from build123d import *

# Parameters (mm, degrees)
EXTRUDE_1_DEPTH      = 406.5
EXTRUDE_1_DEPTH_BACK = 406.5


with BuildPart() as part:
    # 草图1 → 凸台-拉伸1 (new, two sides: drawn at the far end of the back side and taken through both)
    with BuildSketch(Plane.XY.offset(-EXTRUDE_1_DEPTH_BACK)):
        with BuildLine():
            Line((24.75, 1), (24.75, 5.5))
            ThreePointArc((24.75, 5.5), (24.457106781, 6.207106781), (23.75, 6.5))
            Line((23.75, 6.5), (18.5, 6.5))
            Line((18.5, 6.5), (13.25, 6.5))
            ThreePointArc((13.25, 6.5), (12.542893219, 6.207106781), (12.25, 5.5))
            Line((12.25, 5.5), (12.25, 1))
            Line((12.25, 1), (1.35, 1))
            Line((1.35, 1), (1.35, 18))
            ThreePointArc((1.35, 18), (1.935786438, 19.414213562), (3.35, 20))
            Line((3.35, 20), (4.15, 20))
            ThreePointArc((4.15, 20), (4.503553391, 20.146446609), (4.65, 20.5))
            Line((4.65, 20.5), (4.65, 21))
            ThreePointArc((4.65, 21), (4.357106781, 21.707106781), (3.65, 22))
            Line((3.65, 22), (0.05, 22))
            Line((0.05, 22), (0.05, 27.351174762))
            Line((0.05, 27.351174762), (0.25, 27.351174762))
            Line((0.25, 27.351174762), (0.25, 32.3))
            Line((0.25, 32.3), (3.65, 32.3))
            Line((3.65, 32.3), (3.65, 26.3))
            ThreePointArc((3.65, 26.3), (4.15, 25.8), (4.65, 26.3))
            Line((4.65, 26.3), (4.65, 33.8))
            ThreePointArc((4.65, 33.8), (4.503553391, 34.153553391), (4.15, 34.3))
            Line((4.15, 34.3), (-0.35, 34.3))
            ThreePointArc((-0.35, 34.3), (-0.703553391, 34.153553391), (-0.85, 33.8))
            Line((-0.85, 33.8), (-0.85, 27.351174762))
            Line((-0.85, 27.351174762), (-1.35, 27.351174762))
            Line((-1.35, 27.351174762), (-1.35, 20.450932326))
            ThreePointArc((-1.35, 20.450932326), (-0.954594155, 19.496338171), (0, 19.100932326))
            Line((0, 19.100932326), (0, 1))
            ThreePointArc((0, 1), (0.292893219, 0.292893219), (1, 0))
            Line((1, 0), (15.25, 0))
            ThreePointArc((15.25, 0), (15.75, 0.5), (15.25, 1))
            Line((15.25, 1), (13.25, 1))
            Line((13.25, 1), (13.25, 5.5))
            Line((13.25, 5.5), (18.5, 5.5))
            Line((18.5, 5.5), (23.75, 5.5))
            Line((23.75, 5.5), (23.75, 1))
            Line((23.75, 1), (21.75, 1))
            ThreePointArc((21.75, 1), (21.25, 0.5), (21.75, 0))
            Line((21.75, 0), (36, 0))
            ThreePointArc((36, 0), (36.707106781, 0.292893219), (37, 1))
            Line((37, 1), (37, 19.100932326))
            ThreePointArc((37, 19.100932326), (37.954594155, 19.496338171), (38.35, 20.450932326))
            Line((38.35, 20.450932326), (38.35, 27.351174762))
            Line((38.35, 27.351174762), (37.85, 27.351174762))
            Line((37.85, 27.351174762), (37.85, 33.8))
            ThreePointArc((37.85, 33.8), (37.703553391, 34.153553391), (37.35, 34.3))
            Line((37.35, 34.3), (32.85, 34.3))
            ThreePointArc((32.85, 34.3), (32.496446609, 34.153553391), (32.35, 33.8))
            Line((32.35, 33.8), (32.35, 26.3))
            ThreePointArc((32.35, 26.3), (32.85, 25.8), (33.35, 26.3))
            Line((33.35, 26.3), (33.35, 32.3))
            Line((33.35, 32.3), (36.75, 32.3))
            Line((36.75, 32.3), (36.75, 27.351174762))
            Line((36.75, 27.351174762), (36.95, 27.351174762))
            Line((36.95, 27.351174762), (36.95, 22))
            Line((36.95, 22), (33.35, 22))
            ThreePointArc((33.35, 22), (32.642893219, 21.707106781), (32.35, 21))
            Line((32.35, 21), (32.35, 20.5))
            ThreePointArc((32.35, 20.5), (32.496446609, 20.146446609), (32.85, 20))
            Line((32.85, 20), (33.65, 20))
            ThreePointArc((33.65, 20), (35.064213562, 19.414213562), (35.65, 18))
            Line((35.65, 18), (35.65, 1))
            Line((35.65, 1), (24.75, 1))
        make_face()
    extrude(amount=EXTRUDE_1_DEPTH + EXTRUDE_1_DEPTH_BACK)


solid = part.part
The listing builds one solid part. Answer for the finished solid, in the listing's coordinates (mm). A direction names the side the tool comes from. Give positions to 0.01 mm unless a question says otherwise; leave off trailing zeros. Answer as CSV lines item,"result".
Item 1: Given pin 1 Ø4 at (x, z) = (21.5, 150) entering from +Y; pin 2 Ø3 at (x, z) = (18, 6.5) entering from -Y; pin 3 Ø6.5 at (y, z) = (29, 123) entering from -X; pin 4 Ø1 at (y, z) = (29.5, -244.5) entering from -X, each flat-ended and moving along its own axis, determine where each tip first touches the part or whether it passes through.
Values follow:
pin 1,"stops at y = 6.5"
pin 2,"stops at y = 5.5"
pin 3,"stops at x = -1.35"
pin 4,"stops at x = -0.85"
Item 2: The mould has two halves that part along X. Classify faces 1 (the flat face through (29, 0, -6)), 2 (the flat face through (37, 10, -6)), 3 (the flat face through (35.65, 10, -6)): released by +X, released by -X, zero draft, split by the parting line, or undercut.
Values follow:
face 1,"zero draft"
face 2,"released by +X"
face 3,"undercut"
Item 3: Straight lines are drawn through the part: line 1 along Y through (x, z) = (4, -225.5); line 2 along X through (y, z) = (27, -60.5); line 3 along X through (y, z) = (6, 369). For each, find the intervals that lie inside material, in ascending order. Write a range as [from, to].
Values follow:
line 1,"y = [0, 1], [20, 21.94], [25.82, 34.3]"
line 2,"x = [-1.35, 0.05], [3.65, 4.65], [32.35, 33.35], [36.95, 38.35]"
line 3,"x = [0, 1.35], [12.38, 24.62], [35.65, 37]"
Item 4: Which of the six approach directions +Z, -Z, +X, -X, +Y, -Y give full straight-line access (tool end or side, diameter ignored) to faces 4 (the flat face through (0, 10, -6)), 5 (the flat face through (1.35, 9, -6)), 6 (the flat face through (18, 6, 406.5))?
Values follow:
face 4,"+Z, -Z, -X, -Y"
face 5,"+Z, -Z"
face 6,"+Z, +X, -X, +Y, -Y"
